Input: dimensioned drawing with shaded views. Units: mm. Origin: part minimum x, y, z. A direction names the side the tool comes from. Coordinates: 2 decimals unless noted, no trailing zeros.
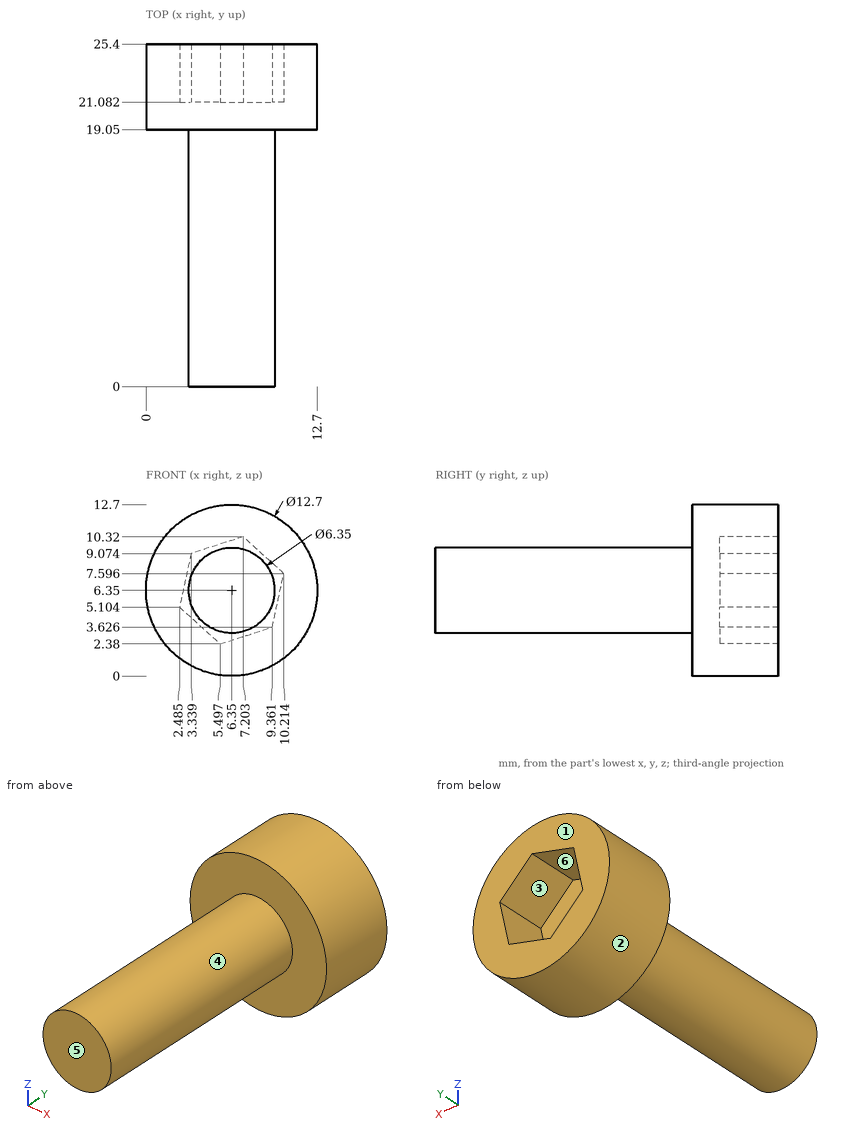
1. Ray query, line 1 (Y direction, x = 4.5, z = 4.25); line 2 (Y direction, x = 3.25, z = 3.25); line 3 (Z direction, x = 6.5, y = 9.75). Return the intervals inside material, ascending.
Findings:
line 1: y = 0 to 21.08
line 2: y = 19.05 to 25.4
line 3: z = 3.18 to 9.52
2. Draft query along Z for the marked faces 1, 2 and 3. Return one class per face: released by +Z, released by -Z, zero draft, split by the parting line, or undercut.
Findings:
face 1: zero draft
face 2: split by the parting line
face 3: undercut
3. Pin query (flat end, axial travel): P1, Ø3, axis at x = 2, y = 9, coming from the +Z side; P2, Ø3, axis at x = 10.5, y = 17.5, coming from the -Z side; P3, Ø4, axis at x = 10, y = 7.5, coming from the +Z side; P4, Ø3, axis at x = 1.5, y = 17.5, coming from the +Z side. Return the tip coordinate at first contact, or that it passes through.
Findings:
P1: stops at z = 7.75
P2: stops at z = 4.6
P3: stops at z = 9.06
P4: passes through
4. Access query for the marked faces 4, 5 and 6. Directions: +Z, -Z, +X, -X, +Y, -Y. A direction counts if a zero-diameter tool reaches every point of the face in a straight line with its end or side. Return the directions, or none.
Findings:
face 4: -Y
face 5: +Z, -Z, +X, -X, -Y
face 6: +Y
